The model under review builds one solid part; all positions refer to its coordinate system, in mm. Face numbers are marked on the shaded views. A direction names the side the tool comes from. Coordinates: 2 decimals unless noted, no trailing zeros. Write each loop counter-clockwise with the first axis right and the second up, starting at its lowest first coordinate (ties: lowest second). Pieces come first, ordered by that corner, then holes. Notation, with made-up numbers: M 46,59 L 71,59 A29 ccw 71,84 Z; hole C 45,18 d3. An arc over 180 degrees is marked long. Answer as a JSON object with one key per item and string values.
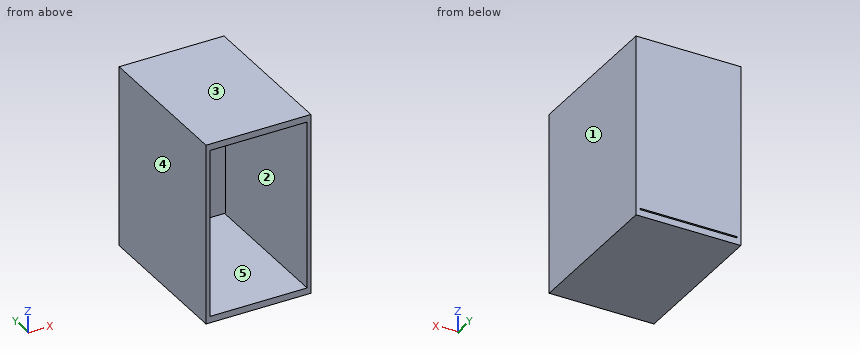
```python
from build123d import *

# Parameters (mm, degrees)
F0_W     = 110
F0_H     = 190
F0_W_2   = 102.098083
F0_H_2   = 176.351235
F1_DEPTH = 160
F2_W     = 103.17653
F2_H     = 175.133594
F3_DEPTH = 10


with BuildPart() as f1:
    # F0 (on Front) → F1 (new body)
    with BuildSketch(Plane.XZ):
        with Locations((-7.087325, -3.817271)):
            Rectangle(F0_W, F0_H)
        with Locations((-7.087326, -3.817271)):
            Rectangle(F0_W_2, F0_H_2, mode=Mode.SUBTRACT)
    extrude(amount=F1_DEPTH)

    # F2 (on Front) → F3 (join)
    with BuildSketch(Plane.XZ):
        with Locations((-7.804865, -3.055822)):
            Rectangle(F2_W, F2_H)
    extrude(amount=F3_DEPTH)


solid = f1.part
```
(1) For pin 1 Ø3 at (x, z) = (-9.5, -77) entering from +Y; pin 2 Ø6 at (x, z) = (-26.5, -61) entering from -Y, all flat-tipped, find the tip position at first contact; note any pin that passes through.
Results list:
{"pin 1": "y = 0", "pin 2": "y = -10"}
(2) Add section B-B on x = -22. Give the boundary of the cut face in (y, z).
Results list:
{"outline": "M -160,-98.82 L 0,-98.82 L 0,-91.99 L -160,-91.99 Z; M -160,84.36 L -10,84.36 L -10,-90.62 L 0,-90.62 L 0,91.18 L -160,91.18 Z"}
(3) Add section A-A on z = 30. Give the boundary of the cut face in (x, y).
Results list:
{"outline": "M -62.09,-160 L -58.14,-160 L -58.14,-10 L 43.78,-10 L 43.78,0 L -62.09,0 Z; M 43.96,-160 L 47.91,-160 L 47.91,0 L 43.96,0 Z"}
(4) Draft analysis for pull direction X (two halves, no side actions). For the marked faces 1, 2 and 3, state which applies: released by +X, released by -X, zero draft, split by the parting line, or undercut.
Results list:
{"face 1": "released by +X", "face 2": "undercut", "face 3": "zero draft"}
(5) Add section C-C on y = -135. Give the boundary of the cut face in (x, z), and give its area (3 significant figures).
Results list:
{"outline": "M -62.09,-98.82 L 47.91,-98.82 L 47.91,91.18 L -62.09,91.18 Z; hole M -58.14,-91.99 L 43.96,-91.99 L 43.96,84.36 L -58.14,84.36 Z", "area": "2,890 mm²"}
(6) Wall thickness on line 1 along Z through (x, y) = (-11.5, -24.5); line 2 along X through (y, z) = (-123.5, -75.5); line 3 along Y through (x, z) = (-58, 33.5): over which ranges is each line inside the solid? List them lowest first. Write a range as from..to.
Results list:
{"line 1": "-98.82..-91.99, 84.36..91.18", "line 2": "-62.09..-58.14, 43.96..47.91", "line 3": "-10..0"}
(7) For the marked faces 4 and 5, list the 3-axis set-ups (+Z, -Z, +X, -X, +Y, -Y) from which the entire face can be reached by the end or side of a thin tool; tool diameter is ignored.
Results list:
{"face 4": "+Z, -Z, -X, +Y, -Y", "face 5": "+Y, -Y"}
